```python
from build123d import *

# Parameters (mm, degrees)
PAD_DEPTH       = 4
SKETCH003_R     = 5.2
POCKET_DEPTH    = 5
FILLET_R        = 5
SKETCH004_R     = 11
PAD001_DEPTH    = 2.5
SKETCH002_R     = 4.5
SKETCH002_R_2   = 1.3
POCKET001_DEPTH = 10
CHAMFER_SIZE    = 1
CHAMFER001_SIZE = 0.2


with BuildPart() as part:
    # Sketch → Pad (new body)
    with BuildSketch(Plane.XY):
        with BuildLine():
            ThreePointArc((-8, 7.549834), (0, -11), (8, 7.549834))
            Line((8, 7.549834), (8, 40))
            Line((8, 40), (-8, 40))
            Line((-8, 40), (-8, 7.549834))
        make_face()
    extrude(amount=PAD_DEPTH)

    # Sketch003 → Pocket (cut)
    with BuildSketch(Plane.XY.offset(4)):
        with Locations((0, 32)):
            Circle(SKETCH003_R)
    extrude(amount=-POCKET_DEPTH, mode=Mode.SUBTRACT)

    # Fillet
    fillet_edges = [part.edges().sort_by_distance(p)[0] for p in [
        (-8, 40, 2),
        (8, 40, 2),
    ]]
    fillet(fillet_edges, radius=FILLET_R)

    # Sketch004 → Pad001 (join)
    with BuildSketch(Plane(origin=(0, 0, 0), x_dir=(1, 0, 0), z_dir=(0, 0, -1))):
        Circle(SKETCH004_R)
    extrude(amount=PAD001_DEPTH)

    # Sketch002 (on Face5 of Pad001) → Pocket001 (cut)
    with BuildSketch(Plane.XY.offset(4)):
        Circle(SKETCH002_R)
        with Locations((0, 8)):
            Circle(SKETCH002_R_2)
        with Locations((5.656854, 5.656854)):
            Circle(SKETCH002_R_2)
        with Locations((8, 0)):
            Circle(SKETCH002_R_2)
        with Locations((5.656854, -5.656854)):
            Circle(SKETCH002_R_2)
        with Locations((0, -8)):
            Circle(SKETCH002_R_2)
        with Locations((-5.656854, -5.656854)):
            Circle(SKETCH002_R_2)
        with Locations((-8, 0)):
            Circle(SKETCH002_R_2)
        with Locations((-5.656854, 5.656854)):
            Circle(SKETCH002_R_2)
    extrude(amount=-POCKET001_DEPTH, mode=Mode.SUBTRACT)

    # Chamfer
    chamfer_edges = [part.edges().sort_by_distance(p)[0] for p in [
        (-6.956854, 5.656854, 4),
        (-1.3, 8, 4),
        (4.356854, 5.656854, 4),
        (6.7, 0, 4),
        (4.356854, -5.656854, 4),
        (-1.3, -8, 4),
        (-6.956854, -5.656854, 4),
        (-9.3, 0, 4),
    ]]
    chamfer(chamfer_edges, length=CHAMFER_SIZE)

    # Chamfer001
    chamfer001_edges = [part.edges().sort_by_distance(p)[0] for p in [
        (-5.2, 32, 4),
        (-4.5, 0, 4),
    ]]
    chamfer(chamfer001_edges, length=CHAMFER001_SIZE)


solid = part.part
```
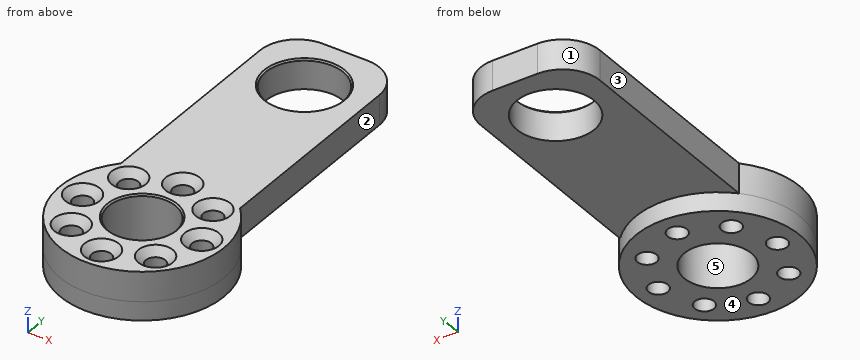
Input: part model. Units: mm. Frame: model coordinates. Face numbers are marked on the shaded views. A direction names the side the tool comes from. Give positions to 0.01 mm unless a question says otherwise; leave off trailing zeros. Order: outer loops, then holes, each group sorted by start corner. A loop starts at its lowest first (then second) coordinate and runs counter-clockwise, first axis right, second up. Notation, with made-up numbers: (-27.5, -33) - (-15.5, -33) arc R24 ccw to (-15.5, -22) - close; hole circle Ø1 at (77, 85.25). An arc over 180 degrees is marked (long way). Put each result on its own line as item: value.
Item 1: Section query C-C, the plane y = 19. Return loops of the section in (x, z).
Found:
outline: (-8, 0) - (8, 0) - (8, 4) - (-8, 4) - close
Item 2: Contact query for flat-ended pins moving along their axis: pin 1 (8 mm diameter, centred on x = 0, y = 0, fed in from +Z); pin 2 (1 mm diameter, centred on x = -8, z = -1.5, fed in from +Y); pin 3 (3 mm diameter, centred on x = 8, y = 0, fed in from +Z); pin 4 (2 mm diameter, centred on y = 9.5, z = 3.5, fed in from +X). Output: stop coordinate, or through.
Found:
pin 1: passes through
pin 2: stops at y = 8.05
pin 3: stops at z = 3.2
pin 4: stops at x = 8
Item 3: Ray query, L1, parallel to Y at x = 0, z = 0.45; L2, parallel to Y at x = 0, z = -0.5; L3, parallel to Y at x = 0.5, z = -0.75. Return the intervals inside material, ascending. Write a range as from..to.
Found:
L1: y = -11..-9.3, -6.7..-4.5, 4.5..6.7, 9.3..26.8, 37.2..40
L2: y = -11..-9.3, -6.7..-4.5, 4.5..6.7, 9.3..11
L3: y = -10.99..-9.2, -6.8..-4.47, 4.47..6.8, 9.2..10.99
Item 4: Draft query along X for the marked faces 3, 4 and 5. Return one class per face: +X half, -X half, draft (parallel to the pull), parting line (faces both ways), or undercut.
Found:
face 3: -X half
face 4: draft
face 5: undercut
Item 5: Section query B-B, the plane z = -1.75. Count the separate pieces of the cut face and the enclosed holes in it, then the cut area to 3 significant figures.
Found:
separate pieces: 1
enclosed holes: 9
area: 274 mm^2
Item 6: Access query for the marked faces 1 and 2. Directions: +Z, -Z, +X, -X, +Y, -Y. A direction counts if a zero-diameter tool reaches every point of the face in a straight line with its end or side. Return the directions, or none.
Found:
face 1: +Z, -Z, -X, +Y
face 2: +Z, -Z, +X, +Y
Item 7: Section query A-A, the plane y = 32. Return loops of the section in (x, z).
Found:
outline: (-8, 0) - (-5.2, 0) - (-5.2, 3.8) - (-5.4, 4) - (-8, 4) - close; (5.2, 0) - (8, 0) - (8, 4) - (5.4, 4) - (5.2, 3.8) - close
